Geometry: final body of the model. Coordinates: model frame, mm. Face numbers are marked on the shaded views. A direction names the side the tool comes from. Give positions to 0.01 mm unless a question says otherwise; leave off trailing zeros. Loops run counter-clockwise (first coordinate to the right, second up) from the corner with the lowest first, then second, coordinate; pieces in that order, holes last.
from build123d import *

# Parameters (mm, degrees)
F1_DEPTH      = 15
F2_W          = 10
F2_H          = 20
F3_DEPTH      = 15.001
F4_R          = 4
F5_DEPTH      = 30.001
F5_DEPTH_BACK = 40.001


with BuildPart() as f1:
    # F0 (on Top) → F1 (new body)
    with BuildSketch(Plane.XY):
        Polygon((-20, 28.8675134595), (-35, 2.8867513459), (-15, -31.7542648054), (15, -31.7542648054), (35, 2.8867513459), (20, 28.8675134595), align=None)
    extrude(amount=F1_DEPTH)

    # F2 (on face) → F3 (cut, through all)
    with BuildSketch(Plane.XY.offset(15)):
        with Locations((0, -31.7542648054)):
            Rectangle(F2_W, F2_H)
        Polygon((-38.6602540378, 16.5470053838), (-21.3397459622, 6.5470053838), (-16.3397459622, 15.2072594216), (-33.6602540378, 25.2072594216), align=None)
        Polygon((33.6602540378, 25.2072594216), (16.3397459622, 15.2072594216), (21.3397459622, 6.5470053838), (38.6602540378, 16.5470053838), align=None)
    extrude(amount=-F3_DEPTH, mode=Mode.SUBTRACT)

    # F4 (on face) → F5 (cut, two sides)
    with BuildSketch(Plane.YZ.offset(-5)) as f5_sk:
        with Locations((-26.7542648054, 7.5)):
            Circle(F4_R)
    extrude(amount=-F5_DEPTH, mode=Mode.SUBTRACT)
    extrude(f5_sk.sketch, amount=F5_DEPTH_BACK, mode=Mode.SUBTRACT)


solid = f1.part
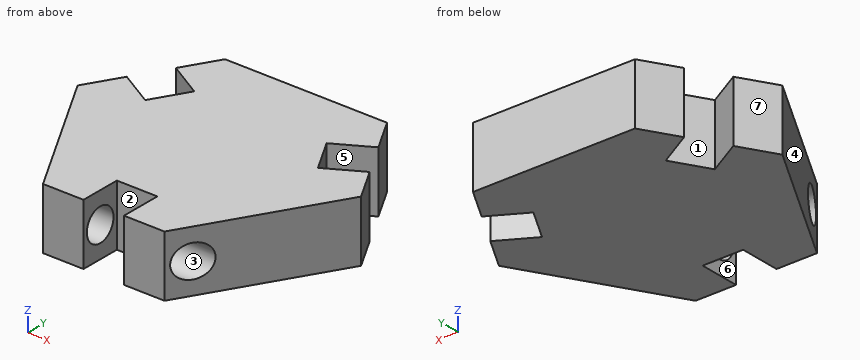
Item 1: Section query B-B on x = -7. Return loops of the section in (y, z).
Values follow:
outline: (-31.75, 0) - (28.87, 0) - (28.87, 15) - (-31.75, 15) - close; hole circle Ø8 at (-26.75, 7.5)
Item 2: Set-up query: the marked faces 1, 2 and 3. Return all of +Z, -Z, +X, -X, +Y, -Y with unobstructed straight access to the full face (end or side cutting, diameter ignored); none if empty.
Values follow:
face 1: +Z, -Z
face 2: +Z, -Z, -Y
face 3: +X, -X
Item 3: Section query A-A on z = 7.5. Return loops of the section in (x, y).
Values follow:
outline: (-35, 2.89) - (-20.2, -22.75) - (-5, -22.75) - (-5, -21.75) - (5, -21.75) - (5, -22.75) - (20.2, -22.75) - (35, 2.89) - (30, 11.55) - (21.34, 6.55) - (16.34, 15.21) - (25, 20.21) - (20, 28.87) - (-20, 28.87) - (-25, 20.21) - (-16.34, 15.21) - (-21.34, 6.55) - (-30, 11.55) - close; (-15.58, -30.75) - (-15, -31.75) - (-5, -31.75) - (-5, -30.75) - close; (5, -31.75) - (15, -31.75) - (15.58, -30.75) - (5, -30.75) - close
Item 4: Ray query, probe 1 along Y at (x, z) = (12.75, 7.5); probe 2 along X at (y, z) = (10, 10); probe 3 along Y at (x, z) = (-15, 5). Return the intervals inside material, ascending.
Values follow:
probe 1: y = -31.75 to -30.75, -22.75 to 28.87
probe 2: x = -30.89 to -27.32, -19.35 to 19.35, 27.32 to 30.89
probe 3: y = -31.75 to -29.88, -23.63 to 28.87
Item 5: Draft query along Y for the marked faces 4, 5, 6 and 7. Return one class per face: +Y half, -Y half, draft (parallel to the pull), parting line (faces both ways), or undercut.
Values follow:
face 4: -Y half
face 5: undercut
face 6: draft
face 7: +Y half
Item 6: Pin query (flat end, axial travel): pin 1 (5 mm diameter, centred on y = -24.5, z = 8.5, fed in from -X); pin 2 (2 mm diameter, centred on y = 5.5, z = 7, fed in from +X); pin 3 (8 mm diameter, centred on y = -4.5, z = 4, fed in from +X). Return the tip coordinate at first contact, or that it passes through.
Values follow:
pin 1: stops at x = -20.63
pin 2: stops at x = 34.07
pin 3: stops at x = 33.04
Item 7: Section query C-C on x = 17.5. Return loops of the section in (y, z), plus the area to 3 significant figures.
Values follow:
outline: (-27.42, 0) - (13.2, 0) - (13.2, 15) - (-27.42, 15) - (-27.42, 11.44) arc R4 cw (long way) to (-27.42, 3.56) - close; (15.88, 0) - (28.87, 0) - (28.87, 15) - (15.88, 15) - close
area: 774 mm2
Item 8: Section query D-D on y = -4. Return loops of the section in (x, z).
Values follow:
outline: (-31.02, 0) - (31.02, 0) - (31.02, 15) - (-31.02, 15) - close
